Design review of the part shown in the three views and the two pictorial views. Dimensions are in mm from the part's minimum x, y and z. Coordinates: 2 decimals unless noted, no trailing zeros. Loops run counter-clockwise (first coordinate to the right, second up) from the corner with the lowest first, then second, coordinate; pieces in that order, holes last. Notation, with made-up numbers: M 76.25,12 L 107.25,12 A9 cw 107.25,27 Z; hole C 42,44.25 d6. An arc over 180 degrees is marked long. Put each result on its own line as item: value. Start each with the question number.
(1) Take a section at B-B, the plane x = 46. Give the boundary of the cut face in (y, z), then the cut area to 3 significant figures.
(2) For probe 1 along Y at (x, z) = (64, 0.8); probe 2 along X at (y, z) = (69.5, 1.25); probe 3 along Z at (x, y) = (36, 51.5), list the stretches that pass through material, from the lowest coordinate up. Write a range as [from, to].
(3) The part is to be moulded in two halves that separate along Y. For the marked faces 1 and 2, say which applies: +Y half, -Y half, draft (parallel to the pull), parting line (faces both ways), or undercut.
(4) Clearance check with a flat-ended pin moving along its axis: pin 1 (19.5 mm diameter, centred on x = 55.5, y = 75.5, fed in from -Z). State where the tip first meets the part, or that it passes through.
(5) Take a section at A-A, the plane y = 79. Give the boundary of the cut face in (x, z).
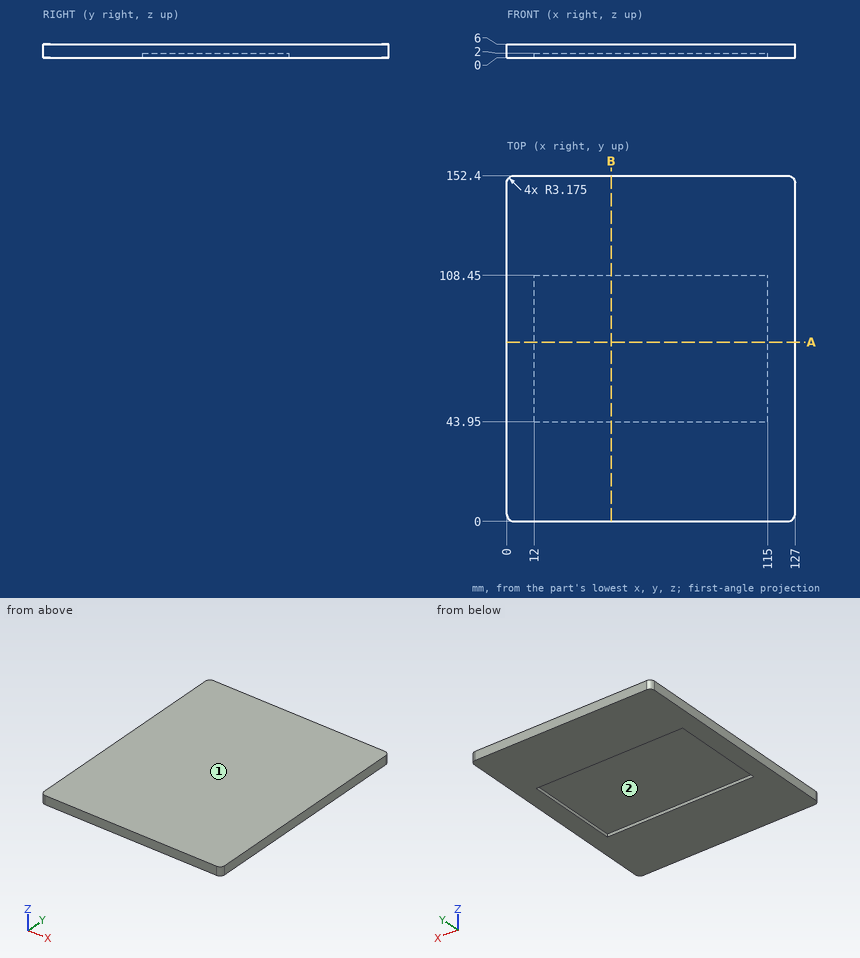
Computed values:
1. outline: M 0,0 L 43.95,0 L 43.95,2 L 108.45,2 L 108.45,0 L 152.4,0 L 152.4,6 L 0,6 Z
1. area: 785 mm^2
2. probe 1: y = [0, 43.95], [108.45, 152.4]
2. probe 2: x = [0, 12], [115, 127]
2. probe 3: z = [2, 6]
3. face 1: draft
3. face 2: undercut
4. pin 1: stops at z = 2
5. outline: M 0,0 L 12,0 L 12,2 L 115,2 L 115,0 L 127,0 L 127,6 L 0,6 Z
